```python
from build123d import *

# Parameters (mm, degrees)
F1_DEPTH = 19.05


with BuildPart() as f1:
    # F0 (on Right) → F1 (new body)
    with BuildSketch(Plane.YZ):
        with BuildLine():
            Line((130.175, -158.75), (130.175, 158.75))
            Line((130.175, 158.75), (12.7, 158.75))
            Line((12.7, 158.75), (12.7, 146.05))
            ThreePointArc((12.7, 146.05), (0, 133.35), (-12.7, 146.05))
            Line((-12.7, 146.05), (-12.7, 158.75))
            Line((-12.7, 158.75), (-130.175, 158.75))
            Line((-130.175, 158.75), (-130.175, -158.75))
            Line((-130.175, -158.75), (130.175, -158.75))
        make_face()
    extrude(amount=F1_DEPTH)


solid = f1.part
```
Read the model definition and answer for the solid it produces. Units are mm, in the model's axes. A direction names the side the tool comes from. Coordinates: 2 decimals unless noted, no trailing zeros. Loops run counter-clockwise (first coordinate to the right, second up) from the corner with the lowest first, then second, coordinate; pieces in that order, holes last.
(1) The mould has two halves that part along Y. Classify faces 1 (the face through (9.392, 0.279, 133.353)), 2 (the face through (9, 72, 158.75)), 3 (the face through (9, 12.7, 152)), 4 (the face through (9, 130.175, -2)): released by +Y, released by -Y, zero draft, split by the parting line, or undercut.
Solution:
face 1: undercut
face 2: zero draft
face 3: undercut
face 4: released by +Y
(2) A tool of negligible diameter and unlimited length cuts with its end or side. For faces 5 (the face through (19.05, -2, 2)), 6 (the face through (9, -12.7, 152)), from which of +Z, -Z, +X, -X, +Y, -Y can it reach the whole face along a straight path? Write none if from no direction.
Solution:
face 5: +Z, -Z, +X, +Y, -Y
face 6: +Z, +X, -X
(3) The part is cut by section A-A (y = 0). Determine the outline of the cut face in (x, z), and give its area (3 significant figures).
Solution:
outline: (0, -158.75) - (19.05, -158.75) - (19.05, 133.35) - (0, 133.35) - close
area: 5,560 mm2
